Verification items for this drawing (mm, ordinates from the low corner). Round coordinates to 2 decimals unless told otherwise and drop trailing zeros. Order: outer loops, then holes, each group sorted by start corner. A loop starts at its lowest first (then second) coordinate and runs counter-clockwise, first axis right, second up. Notation, with made-up numbers: M -10.75,38 L 40.25,38 A13 cw 40.25,45 Z; hole C 66,85 d6. An arc over 180 degrees is marked long. One line per item, written item: value. Start each with the question number.
(1) Cross-section at C-C, the plane x = 10. Enter the section's corners in (y, z).
(2) Cross-section at D-D, the plane z = 15.5. Enter the section's corners in (x, y), and give its area (3 significant figures).
(3) Cross-section at A-A, the plane z = 3. Enter the section's corners in (x, y).
(4) Depth check by flat-ended pin: pin 1 Ø0.8 at (y, z) = (2.5, 10) entering from +X; pin 2 Ø1 at (x, z) = (10, 14) entering from +Y; pin 3 Ø2.5 at (x, z) = (3, 3) entering from +Y; pin 4 Ø0.8 at (x, y) = (10.5, 2.5) entering from +Z. Enter the tip coordinate at first touch or a pass-through.
(5) Thickness scan on L1, parallel to X at y = 1.6, z = 3; L2, parallel to Y at x = 14.75, z = 5.5; L3, parallel to Z at x = 3.25, y = 1. Record the ranges inside material, lowest first.
(6) Cross-section at B-B, the plane x = 3. Enter the section's corners in (y, z).
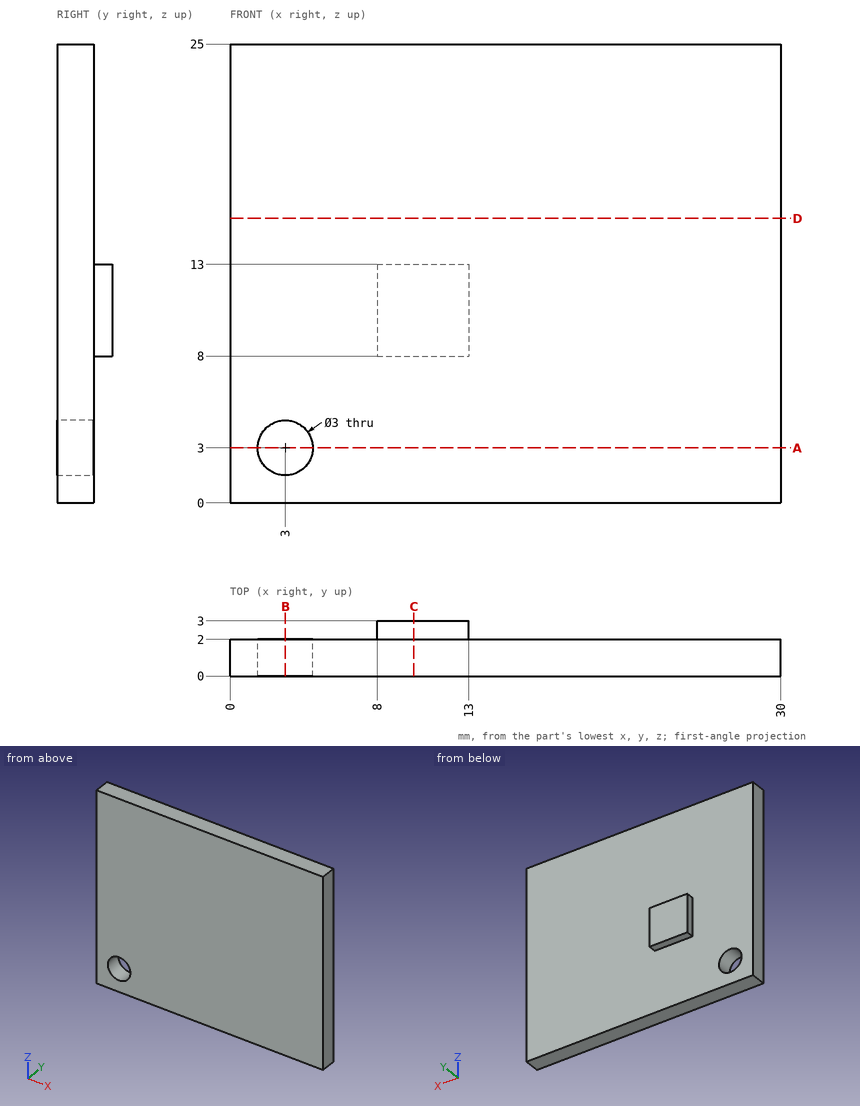
Values found:
1. outline: M 0,0 L 2,0 L 2,8 L 3,8 L 3,13 L 2,13 L 2,25 L 0,25 Z
2. outline: M 0,0 L 30,0 L 30,2 L 0,2 Z
2. area: 60.0 mm^2
3. outline: M 0,0 L 1.5,0 L 1.5,2 L 0,2 Z; M 4.5,0 L 30,0 L 30,2 L 4.5,2 Z
4. pin 1: x = 13
4. pin 2: y = 2
4. pin 3: through
4. pin 4: z = 13
5. L1: 0 to 1.5, 4.5 to 30
5. L2: 0 to 2
5. L3: 0 to 1.52, 4.48 to 25
6. outline: M 0,0 L 2,0 L 2,1.5 L 0,1.5 Z; M 0,4.5 L 2,4.5 L 2,25 L 0,25 Z
